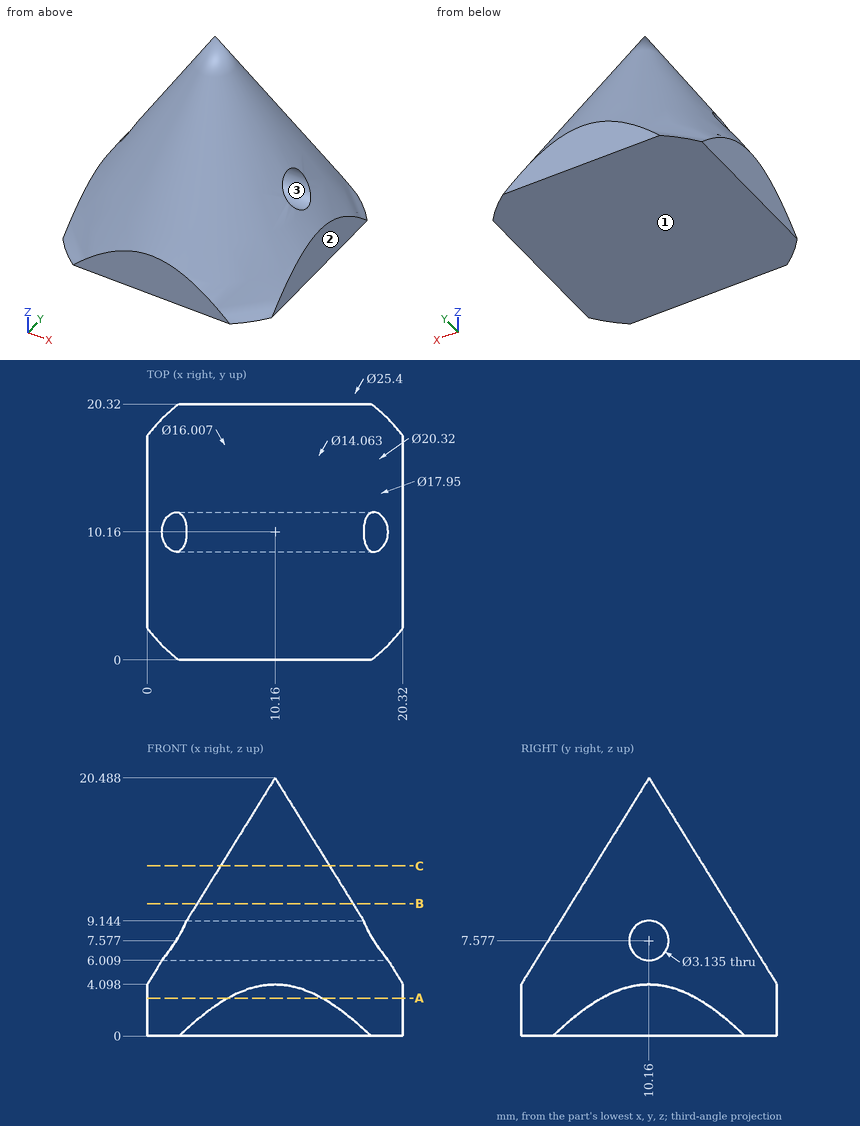
Job drawing, mm, ordinate dimensions from the low corner. One solid piece. Give positions to 0.01 mm unless a question says otherwise; leave off trailing zeros. Write each loop counter-clockwise with the first axis right and the second up, starting at its lowest first coordinate (ties: lowest second). Pieces come first, ordered by that corner, then holes. Notation, with made-up numbers: (57.5, 64) -> (94.5, 64) arc R7 cw to (94.5, 68) -> close; hole circle Ø2 at (46, -34.75). An arc over 180 degrees is marked (long way). Return JSON: item names as keys, results as strings.
Item 1: Band-saw the part on C-C (z = 13.5). List the corners of the cut face in (x, y).
Answer below:
{"outline": "circle Ø8.66 at (10.16, 10.16)"}
Item 2: Band-saw the part on B-B (z = 10.5). List the corners of the cut face in (x, y).
Answer below:
{"outline": "circle Ø12.38 at (10.16, 10.16)"}
Item 3: Drill centre lines: probe 1 along Z at (x, y) = (3.25, 10) (1 decimal); probe 2 along Z at (x, y) = (14.5, 10.16) (1 decimal); probe 3 along Z at (x, y) = (1.75, 5). Where is each one in solid material? Low to high.
Answer below:
{"probe 1": "z = 0 to 6, 9.1 to 9.3", "probe 2": "z = 0 to 6, 9.1 to 13.5", "probe 3": "z = 0 to 4.57"}
Item 4: Drop flat-ended pins along their axis: pin 1 (1.9 mm diameter, centred on y = 10.16, z = 7.58, fed in from -X); pin 2 (3 mm diameter, centred on x = 13.5, z = 7, fed in from +Y); pin 3 (8 mm diameter, centred on y = 7.5, z = 13, fed in from +X); pin 4 (6 mm diameter, centred on x = 16.5, z = 6, fed in from +Y) (1 decimal). Give the stop position or say it passes through.
Answer below:
{"pin 1": "passes through", "pin 2": "stops at y = 18.96", "pin 3": "stops at x = 17.01", "pin 4": "stops at y = 19.6"}
Item 5: Band-saw the part on A-A (z = 3). List the corners of the cut face in (x, y), then the cut area to 3 significant figures.
Answer below:
{"outline": "(0, 6.38) arc R10.84 ccw to (6.38, 0) -> (13.94, 0) arc R10.84 ccw to (20.32, 6.38) -> (20.32, 13.94) arc R10.84 ccw to (13.94, 20.32) -> (6.38, 20.32) arc R10.84 ccw to (0, 13.94) -> close", "area": "355 mm2"}
Item 6: Two-plate mould, pull along Z, no slides. Class the marked faces 1, 2 and 3: +Z half, -Z half, draft (parallel to the pull), parting line (faces both ways), or undercut.
Answer below:
{"face 1": "-Z half", "face 2": "draft", "face 3": "undercut"}
